```python
from build123d import *

# Parameters (mm, degrees)
SKETCH1_W           = 10
SKETCH1_H           = 12
SKETCH2_W           = 2.1
SKETCH2_H           = 4.6
TAPPED_HOLE1_REACH  = 38.29
TAPPED_HOLE1_BORE_R = 1.25
CIRPATTERN1_COUNT   = 2
CIRPATTERN1_ANGLE   = 90
CUT_EXTRUDE1_DEPTH  = 25.738633924


with BuildPart() as part:
    # Sketch1 → Revolve1 (revolve)
    with BuildSketch(Plane.XY, mode=Mode.PRIVATE) as revolve1_sk:
        with Locations((5, 10)):
            Rectangle(SKETCH1_W, SKETCH1_H)
    revolve(revolve1_sk.sketch.rotate(Axis((0, 0, 0), (1, 0, 0)), 180), axis=Axis((0, 0, 0), (1, 0, 0)))

    # Sketch2 → Cut-Revolve1 (revolve, cut)
    with BuildSketch(Plane.XY, mode=Mode.PRIVATE) as cut_revolve1_sk:
        with Locations((6.05, 13.7)):
            Rectangle(SKETCH2_W, SKETCH2_H)
    cut_revolve1 = revolve(cut_revolve1_sk.sketch.rotate(Axis((5, 16, 0), (0, -1, 0)), 180), axis=Axis((5, 16, 0), (0, -1, 0)), mode=Mode.SUBTRACT)

    # Tapped Hole1 bore → Tapped Hole1 (cut, up to next)
    with BuildSketch(Plane(origin=(0, 15, 0), x_dir=(1, 0, 0), z_dir=(0, 1, 0)), mode=Mode.PRIVATE) as tapped_hole1_sk1:
        with Locations((5, 0)):
            Circle(TAPPED_HOLE1_BORE_R)
    tapped_hole1_tool1 = extrude(tapped_hole1_sk1.sketch, amount=-TAPPED_HOLE1_REACH, mode=Mode.PRIVATE) & part.part
    tapped_hole1 = tapped_hole1_tool1.solids().sort_by_distance((5, 15, 0))[0]
    add(tapped_hole1, mode=Mode.SUBTRACT)

    # CirPattern1: Cut-Revolve1, Tapped Hole1 ×2 about axis
    cirpattern1_axis = Axis((0, 0, 0), (-1, 0, 0))
    add([cut_revolve1.rotate(cirpattern1_axis, i * CIRPATTERN1_ANGLE / (CIRPATTERN1_COUNT - 1)) for i in range(1, CIRPATTERN1_COUNT)], mode=Mode.SUBTRACT)
    add([tapped_hole1.rotate(cirpattern1_axis, i * CIRPATTERN1_ANGLE / (CIRPATTERN1_COUNT - 1)) for i in range(1, CIRPATTERN1_COUNT)], mode=Mode.SUBTRACT)

    # Sketch5 → Cut-Extrude1 (cut, through all)
    with BuildSketch(Plane(origin=(0, 0, 0), x_dir=(0, 0, -1), z_dir=(1, 0, 0))):
        with BuildLine():
            Line((-1.5, 0), (1.5, 0))
            Line((1.5, 0), (1.5, 5.2))
            ThreePointArc((1.5, 5.2), (1.441421356, 5.341421356), (1.3, 5.4))
            Line((1.3, 5.4), (-1.3, 5.4))
            ThreePointArc((-1.3, 5.4), (-1.441421356, 5.341421356), (-1.5, 5.2))
            Line((-1.5, 5.2), (-1.5, 0))
        make_face()
    extrude(amount=CUT_EXTRUDE1_DEPTH, mode=Mode.SUBTRACT)

    # Sketch7 → Cut-Revolve3 (revolve, cut)
    with BuildSketch(Plane.XY, mode=Mode.PRIVATE) as cut_revolve3_sk:
        with BuildLine():
            Line((2.113248654, 16), (3.267949192, 14))
            ThreePointArc((3.267949192, 14), (5, 13), (6.732050808, 14))
            Line((6.732050808, 14), (7.886751346, 16))
            Line((7.886751346, 16), (2.113248654, 16))
        make_face()
    revolve(cut_revolve3_sk.sketch.rotate(Axis((0, 0, 0), (1, 0, 0)), 180), axis=Axis((0, 0, 0), (1, 0, 0)), mode=Mode.SUBTRACT)


solid = part.part
```
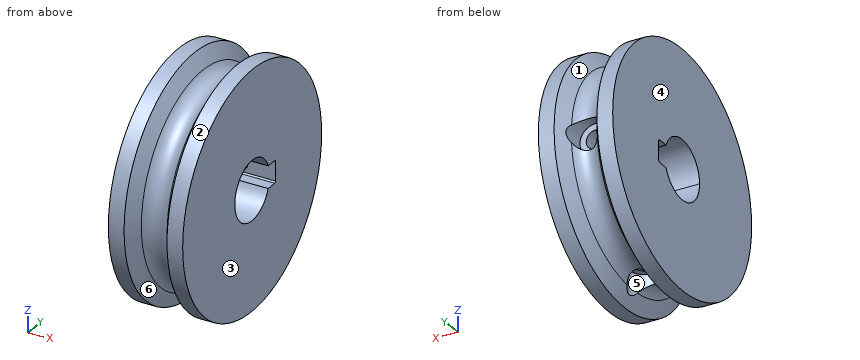
Geometry check sheet. Reference: the model listing, model coordinates, mm. Face numbers are marked on the shaded views. A direction names the side the tool comes from. Give positions to 0.01 mm unless a question says otherwise; leave off trailing zeros. Loops run counter-clockwise (first coordinate to the right, second up) from the corner with the lowest first, then second, coordinate; pieces in that order, holes last. Notation, with made-up numbers: M -38,-32.5 L -25,-32.5 A23 ccw -25,-5.5 Z; hole C -39,22 d5. An arc over 180 degrees is marked long. Answer as CSV lines item,"result".
Item 1: Cross-section at B-B on x = 5. Record the cut outline in (y, z), and give its area (3 significant figures).
Values:
outline,"M -2.1,-12.83 L -2.1,-11.4 L -1.25,-11.4 L -1.25,-3.8 A4 cw long 3.71,1.5 L 5.2,1.5 A0.2 cw 5.4,1.3 L 5.4,1.25 L 11.4,1.25 L 11.4,2.1 L 12.83,2.1 A13 ccw long Z; M 1.25,-11.4 L 2.1,-11.4 L 2.1,-12.83 A13 ccw 12.83,-2.1 L 11.4,-2.1 L 11.4,-1.25 L 5.4,-1.25 L 5.4,-1.3 A0.2 cw 5.2,-1.5 L 3.71,-1.5 A4 cw 1.25,-3.8 Z"
area,"430 mm²"
Item 2: Cross-section at C-C on x = 1.5. Record the cut outline in (y, z), and give its area (3 significant figures).
Values:
outline,"C 0,0 d32; hole M 3.71,-1.5 L 5.2,-1.5 A0.2 ccw 5.4,-1.3 L 5.4,1.3 A0.2 ccw 5.2,1.5 L 3.71,1.5 A4 ccw long Z"
area,"750 mm²"
Item 3: Depth check by flat-ended pin: P1, Ø1, axis at x = 2, z = 1.5, coming from the +Y side; P2, Ø4.5, axis at x = 5, y = 1, coming from the -Z side; P3, Ø4, axis at x = 6, y = 3.5, coming from the +Z side. Enter the tip coordinate at first touch or a pass-through.
Values:
P1,"stops at y = 15.97"
P2,"stops at z = -14.87"
P3,"stops at z = 15.75"
Item 4: Material ranges on line 1 (X direction, y = 10, z = 0); line 2 (Z direction, x = 7.75, y = -2); line 3 (Y direction, x = 5.5, z = -12), recorded low to high.
Values:
line 1,"x = 0 to 3.75, 6.25 to 10"
line 2,"z = -15.64 to -3.46, 3.46 to 15.64"
line 3,"y = -5.16 to -2.04, 2.04 to 5.16"
Item 5: Release check for a two-part mould opening along X. For the marked faces 3, 4, 5 and 6 record: pulls with the +X half, pulls with the -X half, needs draft (parallel to the pull), parting line crosses it, or undercut.
Values:
face 3,"pulls with the +X half"
face 4,"pulls with the -X half"
face 5,"undercut"
face 6,"undercut"
Item 6: Access from +Z, -Z, +X, -X, +Y, -Y to the whole of each face (thin tool, end or side, straight path). Record for the marked faces 1 and 2.
Values:
face 1,"none"
face 2,"+X, -X"
Item 7: Cross-section at A-A on y = 0. Record the cut outline in (x, z), and give its area (3 significant figures).
Values:
outline,"M 0,-16 L 2.11,-16 L 2.9,-14.64 L 2.9,-11.4 L 3.75,-11.4 L 3.75,-4 L 0,-4 Z; M 0,4 L 10,4 L 10,16 L 7.89,16 L 6.73,14 A2 cw 3.27,14 L 2.11,16 L 0,16 Z; M 6.25,-11.4 L 7.1,-11.4 L 7.1,-14.64 L 7.89,-16 L 10,-16 L 10,-4 L 6.25,-4 Z"
area,"189 mm²"
